Source: three-view drawing plus pictorial views. Frame: mm from the lowest corner of the part. A direction names the side the tool comes from. Round coordinates to 2 decimals unless told otherwise and drop trailing zeros. Order: outer loops, then holes, each group sorted by start corner. A loop starts at its lowest first (then second) coordinate and runs counter-clockwise, first axis right, second up. Notation, with made-up numbers: (38, -23) -> (67, -23) arc R17 ccw to (67, -4) -> close; hole circle Ø7 at (70.25, 65). An arc over 180 degrees is marked (long way). Answer as CSV lines item,"result". Start each with the question number.
1) Section query A-A, the plane x = 10. Output: boundary loops of the cut face in (y, z), and give its area (3 significant figures).
2) First-contact query: P1, Ø5, axis at y = 28.5, z = 21.5, coming from the +X side; P2, Ø17, axis at y = 29.5, z = 26, coming from the -X side; P3, Ø5.5, axis at x = 6.5, z = 41, coming from the +Y side. Flat tips, straight axial feed; report the tip coordinate or a pass-through.
3) Section query D-D, the plane y = 50.5. Output: boundary loops of the cut face in (x, z).
4) Line query: L1, parallel to Z at x = 10, y = 7; L2, parallel to Z at x = 25, y = 65.75; L3, parallel to X at y = 65.5, z = 47.4. Output: solid intervals per line, ascending.
5) Section query C-C, the plane x = 44. Output: boundary loops of the cut face in (y, z), and give its area (3 significant figures).
6) Mould query, pull axis Y, two halves, no side actions, for the marked faces 5, 6 and 7. Classes: +Y half, -Y half, draft (parallel to the pull), parting line (faces both ways), or undercut.
7) Access query for the marked faces 1, 2, 3 and 4. Directions: +Z, -Z, +X, -X, +Y, -Y. A direction counts if a zero-diameter tool reaches every point of the face in a straight line with its end or side. Return the directions, or none.
8) Section query B-B, the plane z = 52. Output: boundary loops of the cut face in (x, y), and give its area (3 significant figures).
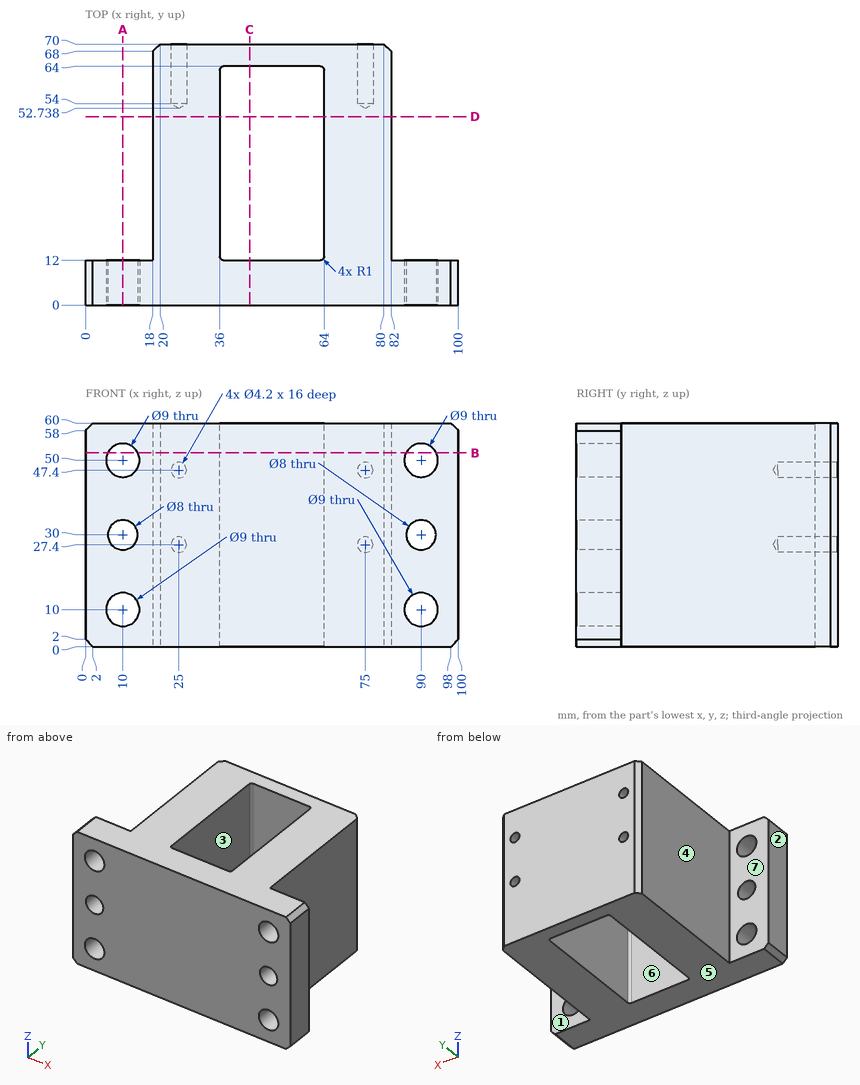
Findings:
1,outline,"(0, 0) -> (12, 0) -> (12, 5.5) -> (0, 5.5) -> close; (0, 14.5) -> (12, 14.5) -> (12, 26) -> (0, 26) -> close; (0, 34) -> (12, 34) -> (12, 45.5) -> (0, 45.5) -> close; (0, 54.5) -> (12, 54.5) -> (12, 60) -> (0, 60) -> close"
1,area,"408 mm^2"
2,P1,"stops at x = 82"
2,P2,"stops at x = 18"
2,P3,"stops at y = 12"
3,outline,"(18, 0) -> (36, 0) -> (36, 60) -> (18, 60) -> close; (64, 0) -> (82, 0) -> (82, 60) -> (64, 60) -> close"
4,L1,"z = 0 to 5.5, 14.5 to 26, 34 to 45.5, 54.5 to 60"
4,L2,"z = 0 to 25.3, 29.5 to 45.3, 49.5 to 60"
4,L3,"x = 18 to 22.9, 27.1 to 72.9, 77.1 to 82"
5,outline,"(0, 0) -> (12, 0) -> (12, 60) -> (0, 60) -> close; (64, 0) -> (70, 0) -> (70, 60) -> (64, 60) -> close"
5,area,"1,080 mm^2"
6,face 5,"draft"
6,face 6,"undercut"
6,face 7,"+Y half"
7,face 1,"+Z, -Z, +X, +Y"
7,face 2,"+Z, -Z, -X, +Y, -Y"
7,face 3,"+Z, -Z"
7,face 4,"+Z, -Z, -X, +Y"
8,outline,"(0, 0) -> (5.97, 0) -> (5.97, 12) -> (0, 12) -> close; (14.03, 0) -> (85.97, 0) -> (85.97, 12) -> (82, 12) -> (82, 68) -> (80, 70) -> (20, 70) -> (18, 68) -> (18, 12) -> (14.03, 12) -> close; (94.03, 0) -> (100, 0) -> (100, 12) -> (94.03, 12) -> close; hole (36, 13) arc R1 ccw to (37, 12) -> (63, 12) arc R1 ccw to (64, 13) -> (64, 63) arc R1 ccw to (63, 64) -> (37, 64) arc R1 ccw to (36, 63) -> close"
8,area,"3,260 mm^2"
